Design review of the part shown in the three views and the two pictorial views. Dimensions are in mm from the part's minimum x, y and z. A direction names the side the tool comes from. Coordinates: 2 decimals unless noted, no trailing zeros. Loops run counter-clockwise (first coordinate to the right, second up) from the corner with the lowest first, then second, coordinate; pieces in that order, holes last. Notation, with made-up numbers: M -12,62.5 L -7,62.5 A29 ccw -7,84.5 Z; hole C -23.75,13 d10. An arc over 180 degrees is marked long. Write item = value, one per line. Start each with the question number.
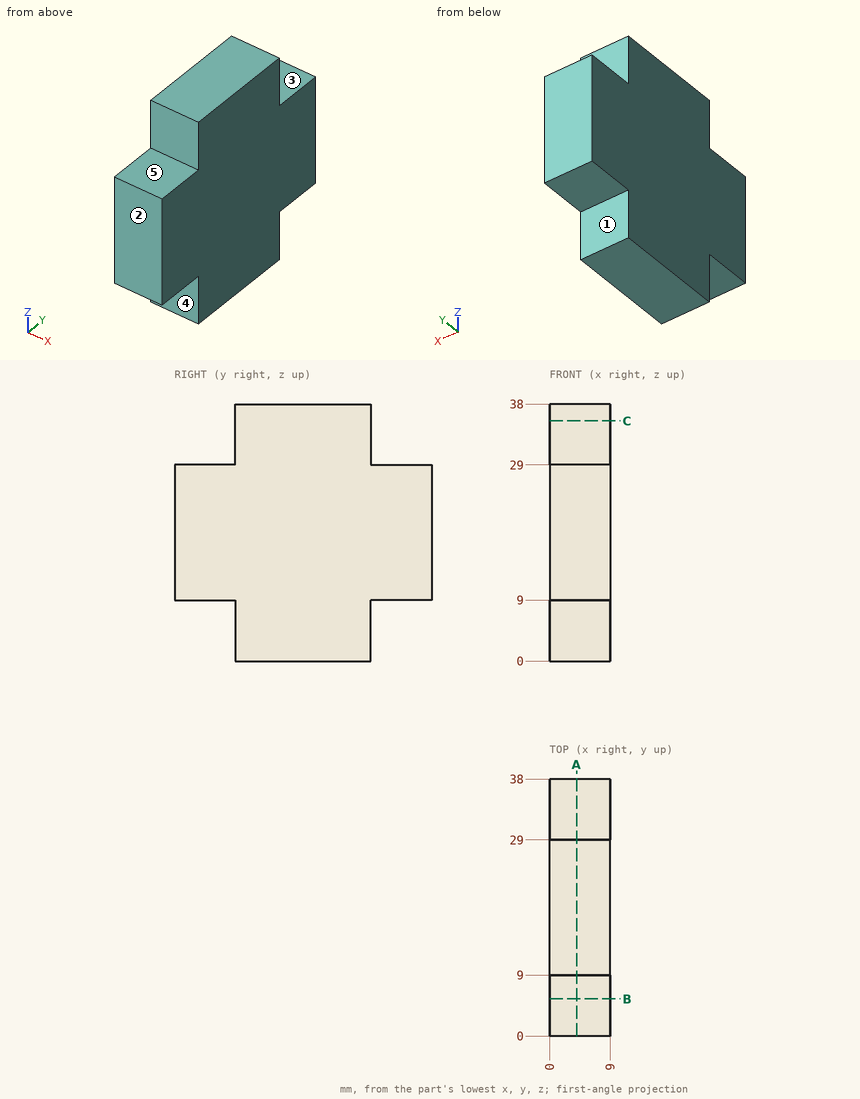
(1) Take a section at B-B (y = 5.5). State the section outline as (x, z) points, plus the area to 3 significant figures.
(2) Insertion check: pin 1 (2.5 mm diameter, centred on x = 4, y = 4.5, fed in from +Z); pin 2 (2.5 mm diameter, centred on x = 5.5, z = 4, fed in from -Y); pin 3 (4.5 mm diameter, centred on x = 4, z = 4, fed in from +Y). Each pin has a flat end and moves straight along its axis. Give the tip position at first contact, or say it passes through.
(3) To check wall thickness, follow L1, parallel to Z at x = 8.5, y = 2. State the ranges of the line that lie inside material, in increasing order.
(4) Take a section at A-A (x = 4). State the section outline as (y, z) points.
(5) Tool access review of the marked faces 1, 2, 3, 4 and 5: name each direction out of +Z, -Z, +X, -X, +Y, -Y from which nothing blocks a thin tool from reaching the whole face with its end or side.
Results list:
q1.outline = M 0,9 L 9,9 L 9,29 L 0,29 Z
q1.area = 180 mm^2
q2.pin_1 = 29
q2.pin_2 = 9
q2.pin_3 = 29
q3.L1 = 9 to 29
q4.outline = M 0,9 L 9,9 L 9,0 L 29,0 L 29,9 L 38,9 L 38,29 L 29,29 L 29,38 L 9,38 L 9,29 L 0,29 Z
q5.face_1 = -Z, +X, -X, +Y
q5.face_2 = +Z, -Z, +X, -X, -Y
q5.face_3 = +Z, +X, -X, +Y
q5.face_4 = -Z, +X, -X, -Y
q5.face_5 = +Z, +X, -X, -Y
